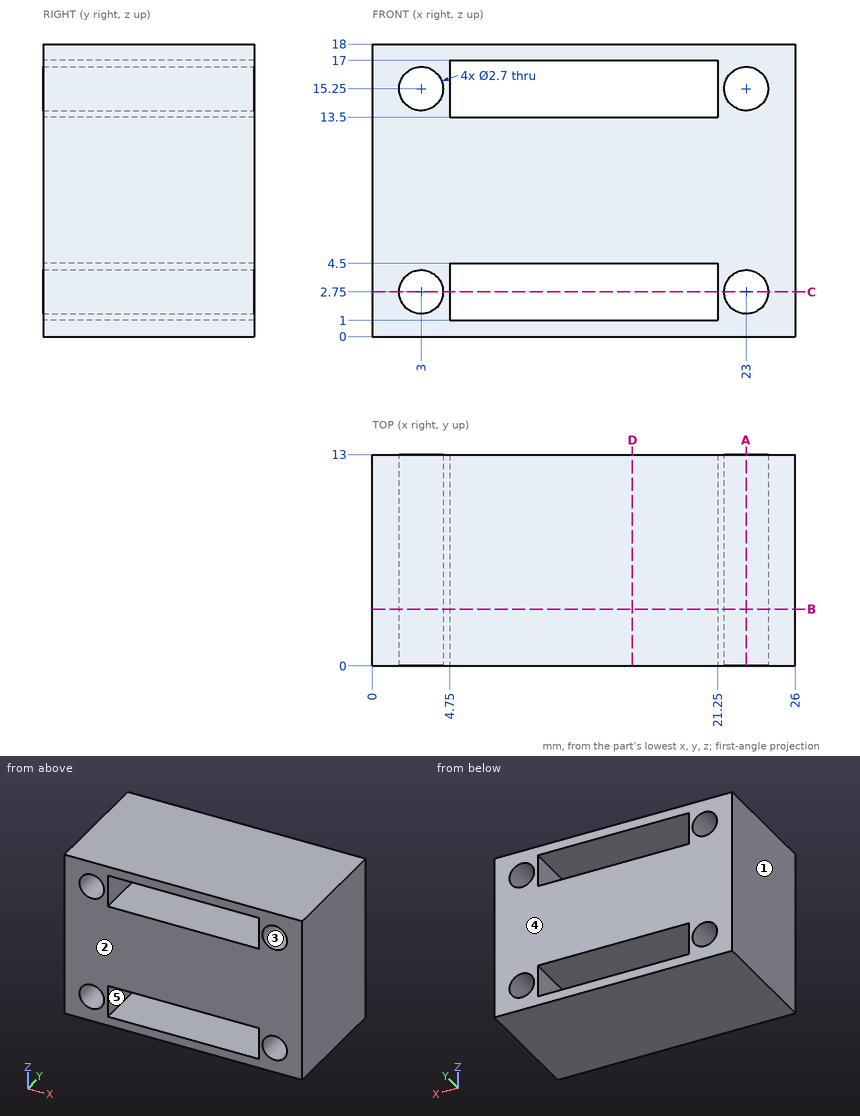
Answer from the drawing. Dimensions are ordinates in mm from the lowest x, y and z of the part. A direction names the side the tool comes from. Round coordinates to 2 decimals unless told otherwise and drop trailing zeros. Loops run counter-clockwise (first coordinate to the right, second up) from the corner with the lowest first, then second, coordinate; pieces in that order, holes last. Notation, with made-up numbers: (15, 30) - (60, 30) arc R31 cw to (60, 63) - close; hole circle Ø4 at (21.25, 25.5). An arc over 180 degrees is marked (long way). Return JSON: item names as keys, results as strings. Group by question number.
1. The part is cut by section C-C on z = 2.75. Determine the outline of the cut face in (x, y).
2. Consider probe 1 along X at (y, z) = (9, 2.75); probe 2 along Z at (x, y) = (3, 7.5); probe 3 along Z at (x, y) = (10.25, 2.75). Determine where each line is inside the solid, lowest interval first.
3. The mould has two halves that part along X. Classify the marked faces 1, 2 and 3: pulls with the +X half, pulls with the -X half, needs draft (parallel to the pull), parting line crosses it, or undercut.
4. Which of the six approach directions +Z, -Z, +X, -X, +Y, -Y give full straight-line access (tool end or side, diameter ignored) to the marked faces 4 and 5?
5. The part is cut by section D-D on x = 16. Determine the outline of the cut face in (y, z).
6. The part is cut by section B-B on y = 3.5. Determine the outline of the cut face in (x, z), then the cut area to 3 significant figures.
7. The part is cut by section A-A on x = 23. Determine the outline of the cut face in (y, z).
Resolved:
{
 "1": {"outline": "(0, 0) - (1.65, 0) - (1.65, 13) - (0, 13) - close; (4.35, 0) - (4.75, 0) - (4.75, 13) - (4.35, 13) - close; (21.25, 0) - (21.65, 0) - (21.65, 13) - (21.25, 13) - close; (24.35, 0) - (26, 0) - (26, 13) - (24.35, 13) - close"},
 "2": {"probe 1": "x = 0 to 1.65, 4.35 to 4.75, 21.25 to 21.65, 24.35 to 26", "probe 2": "z = 0 to 1.4, 4.1 to 13.9, 16.6 to 18", "probe 3": "z = 0 to 1, 4.5 to 13.5, 17 to 18"},
 "3": {"face 1": "pulls with the -X half", "face 2": "needs draft", "face 3": "undercut"},
 "4": {"face 4": "+Z, -Z, +X, -X, +Y", "face 5": "+Y, -Y"},
 "5": {"outline": "(0, 0) - (13, 0) - (13, 1) - (0, 1) - close; (0, 4.5) - (13, 4.5) - (13, 13.5) - (0, 13.5) - close; (0, 17) - (13, 17) - (13, 18) - (0, 18) - close"},
 "6": {"outline": "(0, 0) - (26, 0) - (26, 18) - (0, 18) - close; hole circle Ø2.7 at (3, 2.75); hole circle Ø2.7 at (3, 15.25); hole (4.75, 1) - (21.25, 1) - (21.25, 4.5) - (4.75, 4.5) - close; hole (4.75, 13.5) - (21.25, 13.5) - (21.25, 17) - (4.75, 17) - close; hole circle Ø2.7 at (23, 2.75); hole circle Ø2.7 at (23, 15.25)", "area": "330 mm²"},
 "7": {"outline": "(0, 0) - (13, 0) - (13, 1.4) - (0, 1.4) - close; (0, 4.1) - (13, 4.1) - (13, 13.9) - (0, 13.9) - close; (0, 16.6) - (13, 16.6) - (13, 18) - (0, 18) - close"}
}
